Check sheet for the modelled part. Datum: model origin and axes. Units: mm. A direction names the side the tool comes from. Coordinates: 2 decimals unless noted, no trailing zeros. Loops run counter-clockwise (first coordinate to the right, second up) from the corner with the lowest first, then second, coordinate; pieces in that order, holes last.
```python
from build123d import *

# Parameters (mm, degrees)
F0_W     = 2438.4
F0_H     = 304.8
F0_W_2   = 2400.3
F0_H_2   = 266.7
F1_DEPTH = 254
F2_W     = 2438.4
F2_H     = 304.8
F3_DEPTH = 19.05
F4_W     = 19.05
F4_H     = 266.7
F5_DEPTH = 234.95


with BuildPart() as f1:
    # F0 (on Front) → F1 (new body)
    with BuildSketch(Plane.XZ):
        with Locations((1219.2, -152.4)):
            Rectangle(F0_W, F0_H)
        with Locations((1219.2, -152.4)):
            Rectangle(F0_W_2, F0_H_2, mode=Mode.SUBTRACT)
    extrude(amount=F1_DEPTH)

    # F2 (on Front) → F3 (join)
    with BuildSketch(Plane.XZ):
        with Locations((1219.2, -152.4)):
            Rectangle(F2_W, F2_H)
    extrude(amount=F3_DEPTH)

    # F4 (on face) → F5 (join)
    with BuildSketch(Plane.XZ.offset(19.05)):
        with Locations((1182.107865, -152.4)):
            Rectangle(F4_W, F4_H)
        with Locations((1794.882865, -152.4)):
            Rectangle(F4_W, F4_H)
        with Locations((569.332865, -152.4)):
            Rectangle(F4_W, F4_H)
    extrude(amount=F5_DEPTH)


solid = f1.part
```
1) Scan lines: line 1 (X direction, y = -35, z = -111); line 2 (Z direction, x = 2277.5, y = -163.5); line 3 (Y direction, x = 475.5, z = -97.5). Record each from-to range of solid material in increasing order.
Answer sheet:
line 1: x = 0 to 19.05, 559.81 to 578.86, 1172.58 to 1191.63, 1785.36 to 1804.41, 2419.35 to 2438.4
line 2: z = -304.8 to -285.75, -19.05 to 0
line 3: y = -19.05 to 0
2) Set-up check for faces 5 (the flat face through (0, -125, -155)), 6 (the flat face through (1484, -135, -285.75)): record each of +Z, -Z, +X, -X, +Y, -Y from which the full face is reachable in a straight line by a thin tool's end or side.
Answer sheet:
face 5: +Z, -Z, -X, +Y, -Y
face 6: -Y
3) Section check B-B on x = 907. Enter the section's corners in (y, z), plus the area to 3 significant figures.
Answer sheet:
outline: (-254, -304.8) - (0, -304.8) - (0, 0) - (-254, 0) - (-254, -19.05) - (-19.05, -19.05) - (-19.05, -285.75) - (-254, -285.75) - close
area: 14,800 mm2
4) Depth check by flat-ended pin: pin 1 (3 mm diameter, centred on x = 1225, z = -270.5, fed in from -Y). Enter the tip coordinate at first touch or a pass-through.
Answer sheet:
pin 1: stops at y = -19.05
5) Mould release check, pull along X, two halves, no side actions. Record for faces 1 (the flat face through (2438.4, -125, -155)), 2 (the flat face through (2108, -135, -19.05)), 3 (the flat face through (1202, -125, 0)), 4 (the flat face through (286, -135, -285.75)): +X half, -X half, draft (parallel to the pull), parting line (faces both ways), or undercut.
Answer sheet:
face 1: +X half
face 2: undercut
face 3: draft
face 4: undercut
6) Section check A-A on y = -107.5. Enter the section's corners in (x, z), plus the area to 3 significant figures.
Answer sheet:
outline: (0, -304.8) - (2438.4, -304.8) - (2438.4, 0) - (0, 0) - close; hole (19.05, -285.75) - (559.81, -285.75) - (559.81, -19.05) - (19.05, -19.05) - close; hole (578.86, -285.75) - (1172.58, -285.75) - (1172.58, -19.05) - (578.86, -19.05) - close; hole (1191.63, -285.75) - (1785.36, -285.75) - (1785.36, -19.05) - (1191.63, -19.05) - close; hole (1804.41, -285.75) - (2419.35, -285.75) - (2419.35, -19.05) - (1804.41, -19.05) - close
area: 118,000 mm2
7) Section check C-C on z = -48. Enter the section's corners in (x, y).
Answer sheet:
outline: (0, -254) - (19.05, -254) - (19.05, -19.05) - (559.81, -19.05) - (559.81, -254) - (578.86, -254) - (578.86, -19.05) - (1172.58, -19.05) - (1172.58, -254) - (1191.63, -254) - (1191.63, -19.05) - (1785.36, -19.05) - (1785.36, -254) - (1804.41, -254) - (1804.41, -19.05) - (2419.35, -19.05) - (2419.35, -254) - (2438.4, -254) - (2438.4, 0) - (0, 0) - close
